Geometry: final body of the model. Coordinates: model frame, mm. Give positions to 0.01 mm unless a question says otherwise; leave off trailing zeros. Loops run counter-clockwise (first coordinate to the right, second up) from the corner with the lowest first, then second, coordinate; pieces in that order, holes last. Notation, with made-up numbers: M 84,38.25 L 105,38.25 A18 cw 105,54.25 Z; hole C 53,3 d5. An arc over 180 degrees is marked long. Put each result on its own line as item: value.
Autodesk Inventor part; units mm, degrees
ref_plane "Work Plane1" through (0, 130, 0) normal (0, 1, 0) x (1, 0, 0)
ref_plane "YZ Plane" through (0, 0, 0) normal (1, 0, 0) x (0, 1, 0)
ref_plane "XZ Plane" through (0, 0, 0) normal (0, 1, 0) x (-1, 0, 0)
sketch "Sketch1" plane through (0, 0, 0) normal (0, 1, 0) x (-1, 0, 0)
  line L0 (2.45, -1.4145) -> (0, -2.829)
  line L1 (0, -2.829) -> (-2.45, -1.4145)
  line L2 (-2.45, -1.4145) -> (-2.45, 1.4145)
  line L3 (-2.45, 1.4145) -> (0, 2.829)
  line L4 (0, 2.829) -> (2.45, 1.4145)
  line L5 (2.45, 1.4145) -> (2.45, -1.4145)
  point P0 (0, 0)
  point P1 (0, 0)
  dimension "d0" = 4.9
extrude "Extrusion1" add sketch "Sketch1" along normal blind 120
ref_plane "Work Plane1" through (0, 130, 0) normal (0, 1, 0) x (1, 0, 0)
sketch "Sketch2" plane through (0, 120, 0) normal (0, 1, 0) x (1, 0, 0)
  line L0 (-2.45, 1.4145) -> (0, 2.829)
  line L1 (0, 2.829) -> (2.45, 1.4145)
  line L2 (2.45, 1.4145) -> (2.45, -1.4145)
  line L3 (2.45, -1.4145) -> (0, -2.829)
  line L4 (0, -2.829) -> (-2.45, -1.4145)
  line L5 (-2.45, -1.4145) -> (-2.45, 1.4145)
  point P0 (0, 0)
  point P1 (0, 0)
  dimension "d4" = 4.9
sketch "Sketch3" plane through (0, 130, 0) normal (0, 1, 0) x (1, 0, 0)
  circle A0 centre (0, 0) radius 1
  dimension "d5" = 2
loft "Loft1" add profiles "Sketch3" section 1 edges at (-1.225, 120, -2.1218) (-2.45, 120, 0) (-1.225, 120, 2.1218) (1.225, 120, 2.1218) (2.45, 120, 0) (1.225, 120, -2.1218)
hole "Hole1" at (0, 130, 0) direction (0, -1, 0) diameter 1.5 end through all
properties part number "Pencil Shell"
Item 1: Line query: probe 1 along X at (y, z) = (49.5, -0.55); probe 2 along Z at (x, y) = (0, 50); probe 3 along X at (y, z) = (76, 0). Output: solid intervals per line, ascending. Write a range as [from, to].
Output values:
probe 1: [-2.45, -0.51], [0.51, 2.45]
probe 2: [-2.83, -0.75], [0.75, 2.83]
probe 3: [-2.45, -0.75], [0.75, 2.45]
Item 2: Section A-A on y = 50. Output: boundary loops of the cut face in (x, z).
Output values:
outline: M -2.45,-1.41 L 0,-2.83 L 2.45,-1.41 L 2.45,1.41 L 0,2.83 L -2.45,1.41 Z; hole C 0,0 d1.5
Item 3: Pin query (flat end, axial travel): pin 1 Ø2.5 at (x, z) = (0, 0) entering from -Y; pin 2 Ø1 at (y, z) = (101.5, -2) entering from -X. Return the tip coordinate at first contact, or that it passes through.
Output values:
pin 1: y = 0
pin 2: x = -2.3
